Here's how the part is built. I have some questions about the finished solid (model axes, mm). Face numbers are marked on the shaded views. Give positions to 0.01 mm unless a question says otherwise; leave off trailing zeros. Order: outer loops, then holes, each group sorted by start corner. A loop starts at its lowest first (then second) coordinate and runs counter-clockwise, first axis right, second up. Notation, with made-up numbers: (80.25, 27) - (119.25, 27) arc R20 cw to (119.25, 56) - close; hole circle Ø6 at (29, -10). An arc over 180 degrees is marked (long way). One line per question, with ' | ' between items.
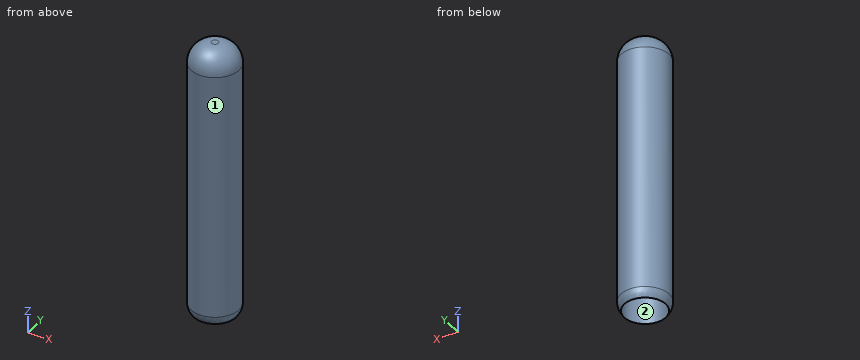
from build123d import *

# Parameters (mm, degrees)
F0_R     = 7
F1_DEPTH = 80
F2_R     = 6
F3_T     = -1


# Not quite as in the source:
# - a fillet or chamfer that OpenCascade refuses, or shapes differently, is made with other operations: its cross-section is extruded or revolved along the edge and cut away or added


with BuildPart() as f1:
    # F0 (on Top) → F1 (new body)
    with BuildSketch(Plane.XY):
        Circle(F0_R)
    extrude(amount=F1_DEPTH)

    # F2
    f2_edges = [f1.edges().sort_by_distance(p)[0] for p in [
        (-7, 0, 80),
    ]]
    fillet(f2_edges, radius=F2_R)

    # F3
    f3_openings = [f1.faces().sort_by_distance(p)[0] for p in [
        (0, 0, 0),
    ]]
    offset(amount=F3_T, openings=f3_openings)

    # F4: fillet of radius 4 on 1 edges, made by hand

    # F4_s1 → F4_t2 (revolve, cut)
    with BuildSketch(Plane.XZ):
        with BuildLine():
            ThreePointArc((7, 2.6457513111), (6.7416573868, 1.2315377487), (6, 0))
            Line((6, 0), (7, 0))
            Line((7, 0), (7, 2.6457513111))
        make_face()
    revolve(axis=Axis((0, 0, 0), (0, 0, 1)), mode=Mode.SUBTRACT)


solid = f1.part
1) Thinking about a two-plate mould opening in X: for the marked faces 1 and 2, which applies, +X half, -X half, draft (parallel to the pull), parting line (faces both ways), or undercut?
Model answer:
face 1: parting line | face 2: undercut
2) I want a section at A-A (z = 6.5). List the corners of the cut face in (x, y) for me, plus the area to 3 significant figures.
Model answer:
outline: circle Ø14 at (0, 0); hole circle Ø12 at (0, 0) | area: 40.8 mm2
3) Please list where these lines run through material, in increasing order: L1, parallel to Y at x = 0, z = 47; L2, parallel to X at y = -0.25, z = 18.5; L3, parallel to X at y = -2.25, z = 54.5.
Model answer:
L1: y = -7 to -6, 6 to 7 | L2: x = -7 to -5.99, 5.99 to 7 | L3: x = -6.63 to -5.56, 5.56 to 6.63
4) I'm going to push flat-ended pins straight in: P1, Ø5, axis at x = -1.5, y = -4.5, coming from the +Z side; P2, Ø3, axis at y = -5, z = 15, coming from the -X side; P3, Ø2, axis at y = -3.5, z = 19.5, coming from the -X side. Where does each tip first touch, or does it pass through?
Model answer:
P1: stops at z = 79.87 | P2: stops at x = -6.06 | P3: stops at x = -6.54
